Verification items for the finished model (mm, model axes). A direction names the side the tool comes from. Round coordinates to 2 decimals unless told otherwise and drop trailing zeros. Loops run counter-clockwise (first coordinate to the right, second up) from the corner with the lowest first, then second, coordinate; pieces in that order, holes last. Notation, with made-up numbers: (-14.75, 58) -> (15.25, 58) arc R12 cw to (15.25, 65) -> close; hole circle Ø2 at (10.5, 0.5). An arc over 180 degrees is marked (long way). Write item = value, one per line. Start each with the question number.
```python
from build123d import *

# Parameters (mm, degrees)
F0_W      = 320
F0_H      = 370
F1_DEPTH  = 63
F2_R      = 20
F3_DEPTH  = 8
F4_R      = 30
F6_W      = 580
F6_H      = 370
F7_DEPTH  = 6
F8_W      = 535
F8_H      = 240
F9_DEPTH  = 189.001
F10_R     = 35
F11_W     = 320
F11_H     = 240
F12_DEPTH = 42
F13_R     = 11
F14_DEPTH = 3
F15_R     = 25
F15_W     = 4
F15_H     = 30
F15_W_2   = 10
F15_H_2   = 12
F16_DEPTH = 3
F15_W_3   = 35
F17_DEPTH = 2.5
F18_R     = 3
F19_DEPTH = 24
F21_W     = 490
F21_H     = 220
F22_DEPTH = 6


with BuildPart() as f1:
    # F0 (on Front) → F1 (new body)
    with BuildSketch(Plane.XZ):
        with Locations((160, 185)):
            Rectangle(F0_W, F0_H)
    extrude(amount=-F1_DEPTH)

    # F2 (on face) → F3 (join)
    with BuildSketch(Plane(origin=(0, 63, 0), x_dir=(-1, 0, 0), z_dir=(0, 1, 0))):
        with Locations((-285, 35)):
            Circle(F2_R)
        with Locations((-285, 335)):
            Circle(F2_R)
        with Locations((-35, 335)):
            Circle(F2_R)
        with Locations((-35, 35)):
            Circle(F2_R)
    extrude(amount=F3_DEPTH)

    # F4
    f4_edges = [f1.edges().sort_by_distance(p)[0] for p in [
        (0, 31.5, 0),
        (320, 31.5, 0),
        (320, 31.5, 370),
        (0, 31.5, 370),
    ]]
    fillet(f4_edges, radius=F4_R)

    # F6 (on line) → F7 (join)
    with BuildSketch(Plane.YZ.offset(189)):
        with Locations((-290, 185)):
            Rectangle(F6_W, F6_H)
    extrude(amount=-F7_DEPTH)

    # F8 (on face) → F9 (cut, through all)
    with BuildSketch(Plane.YZ.offset(189)):
        with Locations((-267.5, 185)):
            Rectangle(F8_W, F8_H)
    extrude(amount=-F9_DEPTH, mode=Mode.SUBTRACT)

    # F10
    f10_edges = [f1.edges().sort_by_distance(p)[0] for p in [
        (186, -580, 0),
        (186, -580, 370),
    ]]
    fillet(f10_edges, radius=F10_R)

    # F11 (on face) → F12 (join)
    with BuildSketch(Plane.XZ):
        with Locations((160, 185)):
            Rectangle(F11_W, F11_H)
    extrude(amount=F12_DEPTH)

    # F13 (on face) → F14 (cut)
    with BuildSketch(Plane.XY.offset(370)):
        with Locations((239, 24)):
            Circle(F13_R)
    extrude(amount=-F14_DEPTH, mode=Mode.SUBTRACT)

    # F15 (on face) → F16 (cut)
    with BuildSketch(Plane(origin=(0, 0, 0), x_dir=(0, -1, 0), z_dir=(-1, 0, 0))):
        with Locations((-32, 101)):
            Circle(F15_R)
        with Locations((-8, 265)):
            Rectangle(F15_W, F15_H)
        with Locations((-31, 265)):
            Rectangle(F15_W_2, F15_H_2)
    extrude(amount=-F16_DEPTH, mode=Mode.SUBTRACT)

    # F15 (on face) → F17 (join)
    with BuildSketch(Plane(origin=(0, 0, 0), x_dir=(0, -1, 0), z_dir=(-1, 0, 0))):
        with Locations((-30.5, 225)):
            Rectangle(F15_W_3, F15_H)
    extrude(amount=F17_DEPTH)

    # F18 (on face) → F19 (join)
    with BuildSketch(Plane.XZ.offset(42)):
        with Locations((30, 95)):
            Circle(F18_R)
        with Locations((30, 275)):
            Circle(F18_R)
        with Locations((290, 95)):
            Circle(F18_R)
        with Locations((290, 275)):
            Circle(F18_R)
    extrude(amount=F19_DEPTH)

    # F21 (on offset) → F22 (join)
    with BuildSketch(Plane.XZ.offset(66)):
        with Locations((165, 185)):
            Rectangle(F21_W, F21_H)
    extrude(amount=F22_DEPTH)


solid = f1.part
```
(1) Access from +Z, -Z, +X, -X, +Y, -Y to the whole of each face (thin tool, end or side, straight path). Record for faces 1 (the flat face through (320, 11, 183)), 2 (the flat face through (90, -21, 65)), 3 (the flat face through (254, 0, 33)).
(2) Scan lines: line 1 (Y direction, x = 210, z = 98); line 2 (Y direction, x = 239, z = 368.8); line 3 (Z direction, x = 2.25, y = 32). Record each from-to range of solid material in increasing order. Write a range as [from, to].
(3) Section check C-C on z = 160. Enter the section's corners in (x, y), then the cut area to 3 significant figures.
(4) Section check B-B on y = -210. Enter the section's corners in (x, z), then the cut area to 3 significant figures.
(5) Section check A-A on x = 102.5. Enter the section's corners in (y, z).
(6) Section check D-D on x = 239. Enter the section's corners in (y, z), then the cut area to 3 significant figures.
(7) Draft check along Z on faces 4 (the cylindrical face through (185.958, -569.475, 9.981)), 5 (the cylindrical face through (266.525, 66.944, 27.34)), 6 (the flat face through (239, 24, 367)), 7 (the flat face through (35, 71, 35)). Enter one of: +Z half, -Z half, draft (parallel to the pull), parting line (faces both ways), or undercut.
(8) Depth check by flat-ended pin: pin 1 Ø1.5 at (x, z) = (14.5, 114.5) entering from +Y; pin 2 Ø1 at (x, z) = (39, 260) entering from -Y; pin 3 Ø3 at (x, y) = (234.5, -68.5) entering from -Z. Enter the tip coordinate at first touch or a pass-through.
Computed values:
q1.face_1 = +Z, -Z, +X, +Y
q1.face_2 = -Z, -X, -Y
q1.face_3 = -Z, +X, -Y
q2.line_1 = [-72, -66], [-42, 63]
q2.line_2 = [0, 13], [35, 63]
q2.line_3 = [18.6, 76], [126, 259], [271, 351.4]
q3.outline = (-80, -72) -> (410, -72) -> (410, -66) -> (-80, -66) -> close; (0, -42) -> (320, -42) -> (320, 63) -> (0, 63) -> close; (183, -580) -> (189, -580) -> (189, -535) -> (183, -535) -> close
q3.area = 36,800 mm²
q4.outline = (183, 0) -> (189, 0) -> (189, 65) -> (183, 65) -> close; (183, 305) -> (189, 305) -> (189, 370) -> (183, 370) -> close
q4.area = 780 mm²
q5.outline = (-72, 75) -> (-66, 75) -> (-66, 295) -> (-72, 295) -> close; (-42, 65) -> (0, 65) -> (0, 0) -> (63, 0) -> (63, 370) -> (0, 370) -> (0, 305) -> (-42, 305) -> close
q6.outline = (-72, 75) -> (-66, 75) -> (-66, 295) -> (-72, 295) -> close; (-42, 65) -> (0, 65) -> (0, 0) -> (63, 0) -> (63, 370) -> (35, 370) -> (35, 367) -> (13, 367) -> (13, 370) -> (0, 370) -> (0, 305) -> (-42, 305) -> close
q6.area = 34,600 mm²
q7.face_4 = -Z half
q7.face_5 = undercut
q7.face_6 = +Z half
q7.face_7 = draft
q8.pin_1 = 63
q8.pin_2 = -72
q8.pin_3 = 75
